Read the model definition and answer for the solid it produces. Units are mm, in the model's axes. Give positions to 0.01 mm unless a question says otherwise; leave off trailing zeros. Loops run counter-clockwise (first coordinate to the right, second up) from the corner with the lowest first, then second, coordinate; pieces in that order, holes last. Notation, with made-up numbers: (65, 40) - (120, 40) arc R15 ccw to (120, 57) - close; hole circle Ø4 at (-36, 20.25). An arc over 180 degrees is marked (long way). Use a Markdown table: item, result. Add a question column.
Item 1: A cutting plane is placed at C-C (y = 80). Determine the outline of the cut face in (x, z) (3 decimals), plus the area to 3 significant figures.
Item 2: A cutting plane is placed at A-A (x = -5.5). Determine the outline of the cut face in (y, z) (3 decimals).
Item 3: Each of these flat-tipped pins is pushed along its axis until it touches: P1, Ø12, axis at x = -17, z = 5.5, coming from the -Y side; P2, Ø5, axis at x = 13, z = -10, coming from the -Y side. Where does it stop, or does it pass through?
Item 4: A cutting plane is placed at B-B (z = -1.75). Determine the outline of the cut face in (x, y) (1 decimal), plus the area to 3 significant figures.
Item 5: Consider probe 1 along Z at (x, y) = (7, 491.5) (3 decimals); probe 2 along X at (y, z) = (102.5, 6.25) (3 decimals); probe 3 along Y at (x, z) = (-2.5, -10). Determine where each line is inside the solid, lowest interval first. Write a range as [from, to].
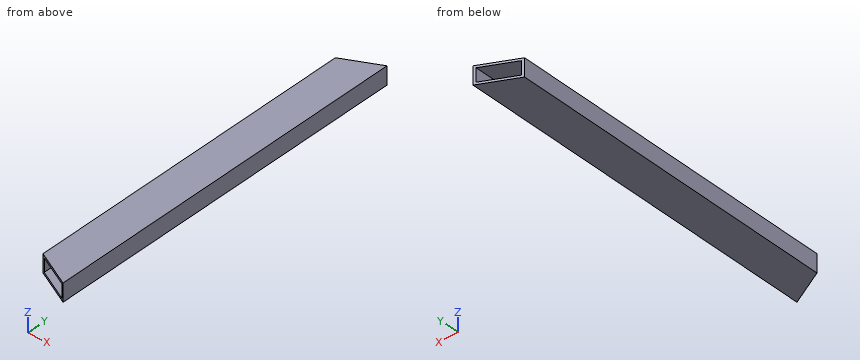
from build123d import *

# Parameters (mm, degrees)
SKETCH1_W           = 50.8
SKETCH1_H           = 25.4
SKETCH1_W_2         = 44.45
SKETCH1_H_2         = 19.05
EXTRUDE_THIN1_DEPTH = 520.7
CUT_EXTRUDE1_DEPTH  = 522.937553736


with BuildPart() as part:
    # Sketch1 → Extrude-Thin1 (new body)
    with BuildSketch(Plane(origin=(0, 0, 0), x_dir=(1, 0, 0), z_dir=(0, 1, 0))):
        Rectangle(SKETCH1_W, SKETCH1_H)
        Rectangle(SKETCH1_W_2, SKETCH1_H_2, mode=Mode.SUBTRACT)
    extrude(amount=EXTRUDE_THIN1_DEPTH)

    # Sketch2 → Cut-Extrude1 (cut, through all)
    with BuildSketch(Plane.XY.offset(12.7)):
        Polygon((25.4, 0), (-25.4, 25.4), (-25.4, 0), align=None)
        Polygon((-25.4, 520.7), (25.4, 520.7), (-25.4, 495.3), align=None)
    extrude(amount=-CUT_EXTRUDE1_DEPTH, mode=Mode.SUBTRACT)


solid = part.part
Geometry says:
| question | item | result |
|---|---|---|
| 1 | outline | (-25.4, -12.7) - (25.4, -12.7) - (25.4, 12.7) - (-25.4, 12.7) - close; hole (-22.225, -9.525) - (22.225, -9.525) - (22.225, 9.525) - (-22.225, 9.525) - close |
| 1 | area | 444 mm² |
| 2 | outline | (15.45, -12.7) - (505.25, -12.7) - (505.25, -9.525) - (15.45, -9.525) - close; (15.45, 9.525) - (505.25, 9.525) - (505.25, 12.7) - (15.45, 12.7) - close |
| 3 | P1 | y = 18.98 |
| 3 | P2 | y = 4.95 |
| 4 | outline | (-25.4, 25.4) - (-22.2, 23.8) - (-22.2, 496.9) - (-25.4, 495.3) - close; (22.2, 1.6) - (25.4, 0) - (25.4, 520.7) - (22.2, 519.1) - close |
| 4 | area | 3,150 mm² |
| 5 | probe 1 | [-12.7, -9.525], [9.525, 12.7] |
| 5 | probe 2 | [-25.4, -22.225], [22.225, 25.4] |
| 5 | probe 3 | [13.95, 506.75] |
